Source: CAD feature listing. Evaluate the final solid. Frame: model axes, mm. Round coordinates to 2 decimals unless told otherwise and drop trailing zeros. Loops run counter-clockwise (first coordinate to the right, second up) from the corner with the lowest first, then second, coordinate; pieces in that order, holes last. Notation, with made-up numbers: (32, -38.75) - (81, -38.75) arc R14 ccw to (81, -19.75) - close; hole circle Ø6 at (0, 69.5). An arc over 180 degrees is marked (long way). One line per question, with ' | ' between items.
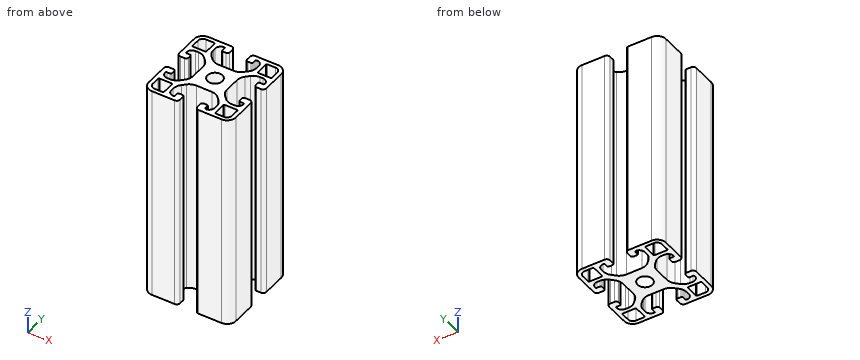
from build123d import *

# Parameters (mm, degrees)
PAD_DEPTH          = 100
POCKET_DEPTH       = 329.783506
POLARPATTERN_COUNT = 4
SKETCH002_R        = 3.4
POCKET001_DEPTH    = 100.001


with BuildPart() as part:
    # Sketch → Pad (new body)
    with BuildSketch(Plane.XY):
        with BuildLine():
            Line((-16, 20), (16, 20))
            ThreePointArc((20, 16), (18.828427, 18.828427), (16, 20))
            Line((20, 16), (20, -16))
            ThreePointArc((16, -20), (18.828427, -18.828427), (20, -16))
            Line((16, -20), (-16, -20))
            ThreePointArc((-20, -16), (-18.828427, -18.828427), (-16, -20))
            Line((-20, -16), (-20, 16))
            ThreePointArc((-16, 20), (-18.828427, 18.828427), (-20, 16))
        make_face()
    extrude(amount=PAD_DEPTH)

    # Sketch001 (on Face10 of Pad) → Pocket (cut, through all)
    with BuildSketch(Plane.XY.offset(100)):
        with BuildLine():
            Line((-16, 18.2), (-12.3, 18.2))
            ThreePointArc((-11.8, 17.7), (-11.946447, 18.053553), (-12.3, 18.2))
            Line((-11.8, 17.7), (-11.8, 12.3))
            ThreePointArc((-12.3, 11.8), (-11.946447, 11.946447), (-11.8, 12.3))
            Line((-12.3, 11.8), (-17.7, 11.8))
            ThreePointArc((-18.2, 12.3), (-18.053553, 11.946447), (-17.7, 11.8))
            Line((-18.2, 12.3), (-18.2, 16))
            ThreePointArc((-16, 18.2), (-17.555635, 17.555635), (-18.2, 16))
        make_face()
        with BuildLine():
            ThreePointArc((-4, 18.5), (-4.43934, 19.56066), (-5.5, 20))
            Line((5.5, 20), (-5.5, 20))
            ThreePointArc((5.5, 20), (4.43934, 19.56066), (4, 18.5))
            Line((4, 16.5), (4, 18.5))
            ThreePointArc((4, 16.5), (4.292893, 15.792893), (5, 15.5))
            Line((6.5, 15.5), (5, 15.5))
            ThreePointArc((6.5, 15.5), (6.853553, 15.646447), (7, 16))
            Line((7, 17.5), (7, 16))
            ThreePointArc((7.5, 18), (7.146447, 17.853553), (7, 17.5))
            ThreePointArc((10, 15.5), (9.267767, 17.267767), (7.5, 18))
            Line((10, 14.19), (10, 15.5))
            ThreePointArc((8.535534, 10.654466), (9.619398, 12.276583), (10, 14.19))
            Line((7.095534, 9.214466), (8.535534, 10.654466))
            ThreePointArc((3.56, 7.75), (5.473417, 8.130602), (7.095534, 9.214466))
            Line((-3.56, 7.75), (3.56, 7.75))
            ThreePointArc((-7.095534, 9.214466), (-5.473417, 8.130602), (-3.56, 7.75))
            Line((-8.535534, 10.654466), (-7.095534, 9.214466))
            ThreePointArc((-10, 14.19), (-9.619398, 12.276583), (-8.535534, 10.654466))
            Line((-10, 15.5), (-10, 14.19))
            ThreePointArc((-7.5, 18), (-9.267767, 17.267767), (-10, 15.5))
            ThreePointArc((-7, 17.5), (-7.146447, 17.853553), (-7.5, 18))
            Line((-7, 16), (-7, 17.5))
            ThreePointArc((-7, 16), (-6.853553, 15.646447), (-6.5, 15.5))
            Line((-5, 15.5), (-6.5, 15.5))
            ThreePointArc((-5, 15.5), (-4.292893, 15.792893), (-4, 16.5))
            Line((-4, 18.5), (-4, 16.5))
        make_face()
    pocket = extrude(amount=-POCKET_DEPTH, mode=Mode.SUBTRACT)

    # PolarPattern: Pocket ×4 about axis
    polarpattern_axis = Axis((0, 0, 100), (0, 0, 1))
    for i in range(1, POLARPATTERN_COUNT):
        add(pocket.rotate(polarpattern_axis, i * 360 / POLARPATTERN_COUNT), mode=Mode.SUBTRACT)

    # Sketch002 (on Face4 of PolarPattern) → Pocket001 (cut, through all)
    with BuildSketch(Plane.XY.offset(100)):
        Circle(SKETCH002_R)
    extrude(amount=-POCKET001_DEPTH, mode=Mode.SUBTRACT)


solid = part.part
1. Material intervals for probe 1 along Y at (x, z) = (-15, 95); probe 2 along Y at (x, z) = (0, 25); probe 3 along Y at (x, z) = (5, 34), sorted ascending.
Worked out:
probe 1: y = -20 to -18.2, -11.8 to -10, 10 to 11.8, 18.2 to 20 | probe 2: y = -7.75 to -3.4, 3.4 to 7.75 | probe 3: y = -19.91 to -15.5, -7.96 to 7.96, 15.5 to 19.91
2. Section query C-C, the plane z = 12.5. Give the number of separate pieces and of enclosed holes in the cut face, plus the area to 3 significant figures.
Worked out:
separate pieces: 1 | enclosed holes: 5 | area: 657 mm2
3. Contact query for flat-ended pins moving along their axis: P1, Ø2, axis at y = -1, z = 26, coming from the -X side; P2, Ø5.5, axis at x = 0.5, z = 28, coming from the -Y side; P3, Ø1, axis at x = -17.5, z = 62, coming from the -Y side; P4, Ø10, axis at x = 4.5, z = 23, coming from the -Y side. Output: stop coordinate, or through.
Worked out:
P1: stops at x = -7.75 | P2: stops at y = -7.75 | P3: stops at y = -19.87 | P4: stops at y = -20
4. Section query A-A, the plane y = 0. Return loops of the section in (x, z), plus the area to 3 significant figures.
Worked out:
outline: (-7.75, 0) - (-3.4, 0) - (-3.4, 100) - (-7.75, 100) - close; (3.4, 0) - (7.75, 0) - (7.75, 100) - (3.4, 100) - close | area: 870 mm2
